Check sheet for the drawn part. Datum: minimum x, y, z corner. Units: mm. Give positions to 0.01 mm unless a question says otherwise; leave off trailing zeros. Loops run counter-clockwise (first coordinate to the right, second up) from the corner with the lowest first, then second, coordinate; pieces in that order, holes last.
1. Cross-section at D-D, the plane y = 0.35. Record the cut outline in (x, z) (1 decimal), plus the area to 3 significant figures.
2. Cross-section at B-B, the plane z = 38.1. Record the cut outline in (x, y) (1 decimal).
3. Cross-section at A-A, the plane x = 12.7. Record the cut outline in (y, z) (1 decimal), plus the area to 3 significant figures.
4. Go/stop test with flat-tipped pins: pin 1 Ø4 at (x, z) = (12.7, 12.7) entering from -Y; pin 2 Ø0.7 at (x, y) = (44, 1) entering from -Z (1 decimal). Record where each tip stops, or that it passes through.
5. Cross-section at C-C, the plane x = 38. Record the cut outline in (y, z) (1 decimal).
6. Material ranges on L1, parallel to Z at x = 12.7, y = 1.7 (1 decimal); L2, parallel to Z at x = 46.5, y = 1.35 (1 decimal); L3, parallel to X at y = 1.4, z = 5, recorded low to high.
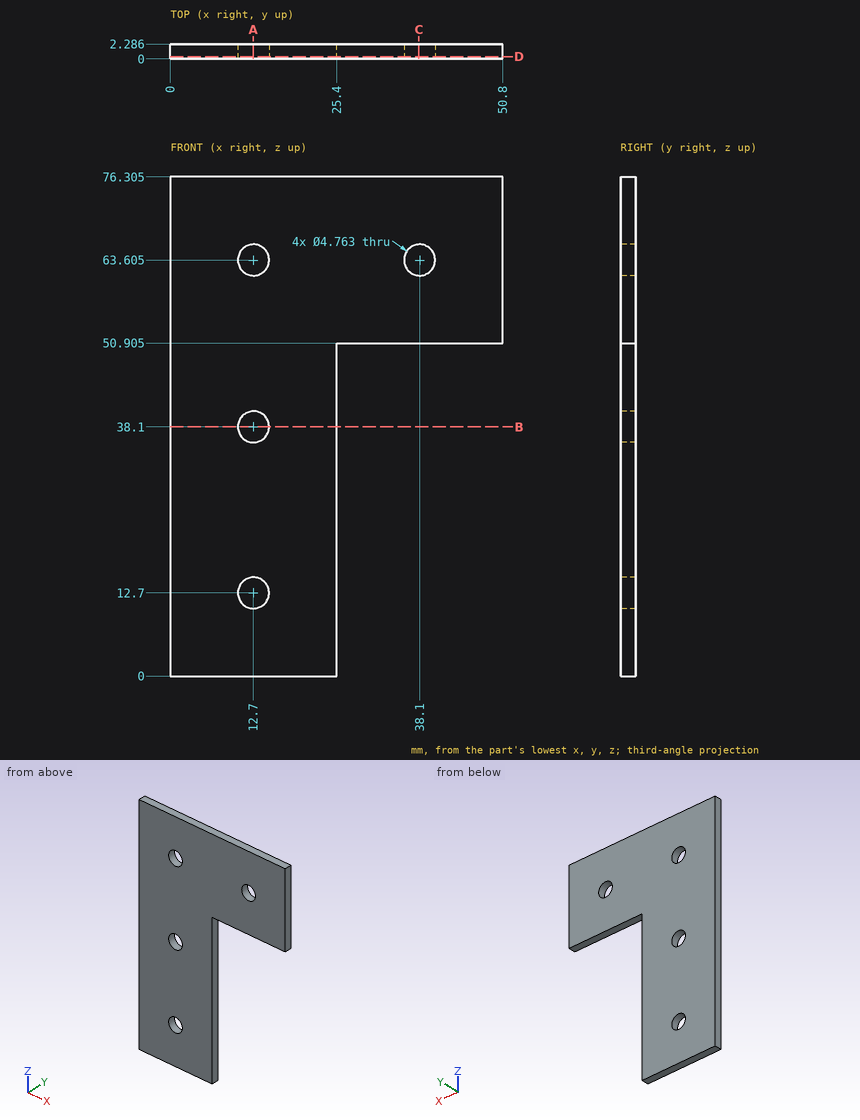
Result:
1. outline: (0, 0) - (25.4, 0) - (25.4, 50.9) - (50.8, 50.9) - (50.8, 76.3) - (0, 76.3) - close; hole circle Ø4.8 at (12.7, 12.7); hole circle Ø4.8 at (12.7, 38.1); hole circle Ø4.8 at (12.7, 63.6); hole circle Ø4.8 at (38.1, 63.6)
1. area: 2,510 mm2
2. outline: (0, 0) - (10.3, 0) - (10.3, 2.3) - (0, 2.3) - close; (15.1, 0) - (25.4, 0) - (25.4, 2.3) - (15.1, 2.3) - close
3. outline: (0, 0) - (2.3, 0) - (2.3, 10.3) - (0, 10.3) - close; (0, 15.1) - (2.3, 15.1) - (2.3, 35.7) - (0, 35.7) - close; (0, 40.5) - (2.3, 40.5) - (2.3, 61.2) - (0, 61.2) - close; (0, 66) - (2.3, 66) - (2.3, 76.3) - (0, 76.3) - close
3. area: 142 mm2
4. pin 1: passes through
4. pin 2: stops at z = 50.9
5. outline: (0, 50.9) - (2.3, 50.9) - (2.3, 61.2) - (0, 61.2) - close; (0, 66) - (2.3, 66) - (2.3, 76.3) - (0, 76.3) - close
6. L1: z = 0 to 10.3, 15.1 to 35.7, 40.5 to 61.2, 66 to 76.3
6. L2: z = 50.9 to 76.3
6. L3: x = 0 to 25.4
